The listing builds one solid part. Answer for the finished solid, in the listing's coordinates (mm). Coordinates: 2 decimals unless noted, no trailing zeros. Order: outer loops, then holes, each group sorted by start corner. A loop starts at its lowest first (then second) coordinate and runs counter-clockwise, first axis right, second up. Notation, with made-up numbers: (84, -19.75) -> (114, -19.75) arc R13 ccw to (114, -8.75) -> close; hole circle Ø3 at (57.5, -30.5). An arc over 180 degrees is marked (long way). Put each result on its own line as item: value. Start each with the question number.
```python
from build123d import *

# Parameters (mm, degrees)
SKETCH1_R               = 11
SKETCH1_R_2             = 10.2
BOSS_EXTRUDE1_DEPTH     = 340.279
CUT_EXTRUDE1_DEPTH      = 378.64
CUT_EXTRUDE1_DEPTH_BACK = 378.64
SKETCH2_R               = 2.756225819
SKETCH2_R_2             = 3.066881292


with BuildPart() as part:
    # Sketch1 → Boss-Extrude1 (new body)
    with BuildSketch(Plane(origin=(0, 0, 0), x_dir=(0, 0, -1), z_dir=(1, 0, 0))):
        Circle(SKETCH1_R)
        Circle(SKETCH1_R_2, mode=Mode.SUBTRACT)
    extrude(amount=BOSS_EXTRUDE1_DEPTH)

    # Sketch2 → Cut-Extrude1 (cut, two sides: drawn at the far end of the back side and taken through both)
    with BuildSketch(Plane.XY.offset(-CUT_EXTRUDE1_DEPTH_BACK)):
        with Locations(Location((21.71, 0, 0), (0, 0, 180))):
            Circle(SKETCH2_R)
        with Locations(Location((297.279, 0, 0), (0, 0, 180))):
            Circle(SKETCH2_R_2)
    extrude(amount=CUT_EXTRUDE1_DEPTH + CUT_EXTRUDE1_DEPTH_BACK, mode=Mode.SUBTRACT)


solid = part.part
```
(1) Each of these flat-tipped pins is pushed along its axis until it touches: P1, Ø1.5, axis at x = 177, z = -7.5, coming from the +Y side; P2, Ø1, axis at x = 200.5, z = 1.5, coming from the +Y side; P3, Ø8, axis at x = 195.5, z = 4.5, coming from the -Y side. Where does it stop, or does it pass through?
(2) Find the intervals of material crossed by L1, parallel to Z at x = 125, y = 0; L2, parallel to Z at x = 202, y = 2.5, in increasing order.
(3) The part is cut by section C-C on x = 21.71. Determine the outline of the cut face in (y, z).
(4) For a pull along Y with two mould halves and no side action, classify faces 1 (the flat face through (340.279, -10, -3)), 2 (the cylindrical face through (167.76, -10.74, 2.38)), 3 (the cylindrical face through (300.343, -0.135, -10.373)) as released by +Y, released by -Y, zero draft, split by the parting line, or undercut.
(5) The part is cut by section D-D on x = 154.5. Determine the outline of the cut face in (y, z), plus the area to 3 significant figures.
(6) The part is cut by section B-B on z = 0. Determine the outline of the cut face in (x, y), plus the area to 3 significant figures.
(7) The part is cut by section A-A on y = 0. Determine the outline of the cut face in (x, z).
Worked out:
1. P1: y = 8.69
1. P2: y = 10.95
1. P3: y = -10.99
2. L1: -11 to -10.2, 10.2 to 11
2. L2: -10.71 to -9.89, 9.89 to 10.71
3. outline: (-2.76, -10.65) -> (-2.76, -9.82) arc R10.2 cw to (-2.76, 9.82) -> (-2.76, 10.65) arc R11 ccw to start; (2.76, -10.65) arc R11 ccw to (2.76, 10.65) -> (2.76, 9.82) arc R10.2 cw to (2.76, -9.82) -> close
4. face 1: zero draft
4. face 2: split by the parting line
4. face 3: undercut
5. outline: circle Ø22 at (0, 0); hole circle Ø20.4 at (0, 0)
5. area: 53.3 mm2
6. outline: (0, -11) -> (340.28, -11) -> (340.28, -10.2) -> (0, -10.2) -> close; (0, 10.2) -> (340.28, 10.2) -> (340.28, 11) -> (0, 11) -> close
6. area: 544 mm2
7. outline: (0, -11) -> (18.95, -11) -> (18.95, -10.2) -> (0, -10.2) -> close; (0, 10.2) -> (18.95, 10.2) -> (18.95, 11) -> (0, 11) -> close; (24.47, -11) -> (294.21, -11) -> (294.21, -10.2) -> (24.47, -10.2) -> close; (24.47, 10.2) -> (294.21, 10.2) -> (294.21, 11) -> (24.47, 11) -> close; (300.35, -11) -> (340.28, -11) -> (340.28, -10.2) -> (300.35, -10.2) -> close; (300.35, 10.2) -> (340.28, 10.2) -> (340.28, 11) -> (300.35, 11) -> close
